Geometry check sheet. Reference: the model listing, model coordinates, mm. A direction names the side the tool comes from. Round coordinates to 2 decimals unless told otherwise and drop trailing zeros. Loops run counter-clockwise (first coordinate to the right, second up) from the corner with the lowest first, then second, coordinate; pieces in that order, holes last. Notation, with made-up numbers: (-32, -6.5) - (-13, -6.5) arc R15 cw to (-13, 19.5) - close; hole circle Ø9 at (-25, 67). An arc over 180 degrees is marked (long way). Answer in a Markdown table with one row per item. Add a question column.
```python
from build123d import *

# Parameters (mm, degrees)
S01_PRINTABLE_SLIDING_PIN_7_90_MM_R            = 3.95
F_01_PRINTABLE_SLIDING_PIN_7_90_MM_DEPTH       = 40
F_02_START                                     = 40
S02_RECESSED_LOAD_SHOULDER_R                   = 5.25
F_02_RECESSED_LOAD_SHOULDER_DEPTH              = 2
F_03_START                                     = 42
S03_LOCATING_PILOT_THROUGH_SWING_ARM_R         = 4
F_03_LOCATING_PILOT_THROUGH_SWING_ARM_DEPTH    = 7.8
F_04_START                                     = 42.6
S04_M3_HEAT_SET_POCKET_IN_SUPPORTED_RO_R       = 2
F_04_M3_HEAT_SET_POCKET_IN_SUPPORTED_ROO_DEPTH = 7.3


with BuildPart() as part:
    # S01 - Printable sliding pin - 7.90 mm → 01 - Printable sliding pin - 7.90 mm (new body)
    with BuildSketch(Plane.XY):
        Circle(S01_PRINTABLE_SLIDING_PIN_7_90_MM_R)
    extrude(amount=F_01_PRINTABLE_SLIDING_PIN_7_90_MM_DEPTH)

    # S02 - Recessed load shoulder → 02 - Recessed load shoulder (add)
    with BuildSketch(Plane.XY.offset(F_02_START)):
        Circle(S02_RECESSED_LOAD_SHOULDER_R)
    extrude(amount=F_02_RECESSED_LOAD_SHOULDER_DEPTH)

    # S03 - Locating pilot through swing arm → 03 - Locating pilot through swing arm (add)
    with BuildSketch(Plane.XY.offset(F_03_START)):
        Circle(S03_LOCATING_PILOT_THROUGH_SWING_ARM_R)
    extrude(amount=F_03_LOCATING_PILOT_THROUGH_SWING_ARM_DEPTH)

    # S04 - M3 heat-set pocket in supported root → 04 - M3 heat-set pocket in supported root (cut)
    with BuildSketch(Plane.XY.offset(F_04_START)):
        Circle(S04_M3_HEAT_SET_POCKET_IN_SUPPORTED_RO_R)
    extrude(amount=F_04_M3_HEAT_SET_POCKET_IN_SUPPORTED_ROO_DEPTH, mode=Mode.SUBTRACT)


solid = part.part
```
Q1. Cross-section at C-C, the plane z = 46.5. Enter the section's corners in (x, y).
Q2. Cross-section at D-D, the plane z = 10. Enter the section's corners in (x, y).
Q3. Release check for a two-part mould opening along Y. For faces 4 (the cylindrical face through (0, -2, 46)), 5 (the flat face through (0, 0, 42.6)), 6 (the cylindrical face through (-3.135, -2.404, 19.72)), 7 (the flat face through (-2, -1, 49.8)) record: +Y half, -Y half, draft (parallel to the pull), parting line (faces both ways), or undercut.
Q4. Scan lines: line 1 (Y direction, x = 0, z = 45.5); line 2 (X direction, y = -0.25, z = 42.5); line 3 (Y direction, x = 0, z = 22.5). Record each from-to range of solid material in increasing order. Write a range as from..to.
Q5. Cross-section at A-A, the plane y = 0. Enter the section's corners in (x, z), plus the area to 3 significant figures.
Q6. Set-up check for faces 1 (the cylindrical face through (5, 1.6, 41)), 2 (the cylindrical face through (-0.867, -3.905, 45.845)), 3 (the flat face through (1, 4, 40)): record each of +Z, -Z, +X, -X, +Y, -Y from which the full face is reachable in a straight line by a thin tool's end or side.
Q7. Depth check by flat-ended pin: P1, Ø6, axis at x = 3, z = 31.5, coming from the -Y side; P2, Ø1, axis at y = -2.5, z = 26, coming from the +X side; P3, Ø2, axis at y = -2, z = 22, coming from the +X side. Enter the tip coordinate at first touch or a pass-through.
Check sheet entries:
| question | item | result |
|---|---|---|
| 1 | outline | circle Ø8 at (0, 0); hole circle Ø4 at (0, 0) |
| 2 | outline | circle Ø7.9 at (0, 0) |
| 3 | face 4 | undercut |
| 3 | face 5 | undercut |
| 3 | face 6 | parting line |
| 3 | face 7 | draft |
| 4 | line 1 | -4..-2, 2..4 |
| 4 | line 2 | -3.99..3.99 |
| 4 | line 3 | -3.95..3.95 |
| 5 | outline | (-5.25, 40) - (-3.95, 40) - (-3.95, 0) - (3.95, 0) - (3.95, 40) - (5.25, 40) - (5.25, 42) - (4, 42) - (4, 49.8) - (2, 49.8) - (2, 42.6) - (-2, 42.6) - (-2, 49.8) - (-4, 49.8) - (-4, 42) - (-5.25, 42) - close |
| 5 | area | 371 mm² |
| 6 | face 1 | +Z, -Z |
| 6 | face 2 | +Z |
| 6 | face 3 | -Z |
| 7 | P1 | y = -3.95 |
| 7 | P2 | x = 3.41 |
| 7 | P3 | x = 3.82 |
